The model under review builds one solid part; all positions refer to its coordinate system, in mm. A direction names the side the tool comes from. Give positions to 0.01 mm unless a question says otherwise; leave off trailing zeros. Loops run counter-clockwise (first coordinate to the right, second up) from the corner with the lowest first, then second, coordinate; pieces in that order, holes last. Notation, with made-up numbers: M 16.25,64.5 L 63.25,64.5 A32 ccw 63.25,103.5 Z; hole C 15,61 d11. An arc over 180 degrees is marked long. Put each result on its own line as item: value. Start each with the question number.
from build123d import *

# Parameters (mm, degrees)
SKETCH_1_W                        = 635
SKETCH_1_H                        = 803
SM_BASE_FLANGE_1_DEPTH            = 1
SM_EDGE_FLANGE_1_STRIP_W          = 5.4732
SM_EDGE_FLANGE_1_STRIP_H          = 1
SM_EDGE_FLANGE_1_STRIP_CUT_DEPTH  = 535
SM_EDGE_FLANGE_1_RELIEF_W         = 5.9732
SM_EDGE_FLANGE_1_RELIEF_H         = 0.5
SM_EDGE_FLANGE_1_RELIEF_CUT_DEPTH = 1
SM_EDGE_FLANGE_1_DEPTH            = 535
SM_EDGE_FLANGE_2_STRIP_W          = 5.4732
SM_EDGE_FLANGE_2_STRIP_H          = 1
SM_EDGE_FLANGE_2_STRIP_CUT_DEPTH  = 535
SM_EDGE_FLANGE_2_RELIEF_W         = 5.9732
SM_EDGE_FLANGE_2_RELIEF_H         = 0.5
SM_EDGE_FLANGE_2_RELIEF_CUT_DEPTH = 1
SM_EDGE_FLANGE_2_DEPTH            = 535
SM_EDGE_FLANGE_3_STRIP_W          = 5.4732
SM_EDGE_FLANGE_3_STRIP_H          = 1
SM_EDGE_FLANGE_3_STRIP_CUT_DEPTH  = 703
SM_EDGE_FLANGE_3_RELIEF_W         = 5.9732
SM_EDGE_FLANGE_3_RELIEF_H         = 0.5
SM_EDGE_FLANGE_3_RELIEF_CUT_DEPTH = 1
SM_EDGE_FLANGE_3_DEPTH            = 703
SM_EDGE_FLANGE_3_FLAT_DEPTH       = 1
SKETCH_15_R                       = 3
CUT_EXTRUDE_2_DEPTH               = 752.549898543
SKETCH_16_R                       = 3
CUT_EXTRUDE_3_DEPTH               = 513.258235659


# Sheet-metal steps are written as plain solids
with BuildPart() as part:
    # Sketch 1 → 基体-法兰1 (new body)
    with BuildSketch(Plane.XY):
        Rectangle(SKETCH_1_W, SKETCH_1_H)
    extrude(amount=-SM_BASE_FLANGE_1_DEPTH)

    # 边线-法兰1 strip (across the edge) → 边线-法兰1 strip cut (cut)
    with BuildSketch(Plane(origin=(-267.5, 401.5, -1), x_dir=(0, -1, 0), z_dir=(1, 0, 0))):
        with Locations((-1, -0.5)):
            Rectangle(SM_EDGE_FLANGE_1_STRIP_W, SM_EDGE_FLANGE_1_STRIP_H)
    extrude(amount=SM_EDGE_FLANGE_1_STRIP_CUT_DEPTH, mode=Mode.SUBTRACT)

    # 边线-法兰1 relief (on the sheet) → 边线-法兰1 relief cut (cut)
    with BuildSketch(Plane(origin=(-267.5, 399.7634, -1), x_dir=(0, -1, 0), z_dir=(0, 0, -1))):
        with Locations((-2.4866, 0.25)):
            Rectangle(SM_EDGE_FLANGE_1_RELIEF_W, SM_EDGE_FLANGE_1_RELIEF_H)
        with Locations((-2.4866, -535.25)):
            Rectangle(SM_EDGE_FLANGE_1_RELIEF_W, SM_EDGE_FLANGE_1_RELIEF_H)
    extrude(amount=-SM_EDGE_FLANGE_1_RELIEF_CUT_DEPTH, mode=Mode.SUBTRACT)

    # 边线-法兰1 section (across the edge) → 边线-法兰1 (add)
    with BuildSketch(Plane(origin=(-267.5, 401.5, -1), x_dir=(0, -1, 0), z_dir=(1, 0, 0))):
        with BuildLine():
            Line((0, 0.7366), (0, 19))
            Line((0, 19), (1, 19))
            Line((1, 19), (1, 0.7366))
            ThreePointArc((1, 0.7366), (1.215745145, 0.215745145), (1.7366, 0))
            Line((1.7366, 0), (1.7366, -1))
            ThreePointArc((1.7366, -1), (0.508638364, -0.491361636), (0, 0.7366))
        make_face()
    extrude(amount=SM_EDGE_FLANGE_1_DEPTH)

    # 边线-法兰2 strip (across the edge) → 边线-法兰2 strip cut (cut)
    with BuildSketch(Plane(origin=(267.5, -401.5, -1), x_dir=(0, 1, 0), z_dir=(-1, 0, 0))):
        with Locations((-1, -0.5)):
            Rectangle(SM_EDGE_FLANGE_2_STRIP_W, SM_EDGE_FLANGE_2_STRIP_H)
    extrude(amount=SM_EDGE_FLANGE_2_STRIP_CUT_DEPTH, mode=Mode.SUBTRACT)

    # 边线-法兰2 relief (on the sheet) → 边线-法兰2 relief cut (cut)
    with BuildSketch(Plane(origin=(267.5, -399.7634, -1), x_dir=(0, 1, 0), z_dir=(0, 0, -1))):
        with Locations((-2.4866, 0.25)):
            Rectangle(SM_EDGE_FLANGE_2_RELIEF_W, SM_EDGE_FLANGE_2_RELIEF_H)
        with Locations((-2.4866, -535.25)):
            Rectangle(SM_EDGE_FLANGE_2_RELIEF_W, SM_EDGE_FLANGE_2_RELIEF_H)
    extrude(amount=-SM_EDGE_FLANGE_2_RELIEF_CUT_DEPTH, mode=Mode.SUBTRACT)

    # 边线-法兰2 section (across the edge) → 边线-法兰2 (add)
    with BuildSketch(Plane(origin=(267.5, -401.5, -1), x_dir=(0, 1, 0), z_dir=(-1, 0, 0))):
        with BuildLine():
            Line((0, 0.7366), (0, 19))
            Line((0, 19), (1, 19))
            Line((1, 19), (1, 0.7366))
            ThreePointArc((1, 0.7366), (1.215745145, 0.215745145), (1.7366, 0))
            Line((1.7366, 0), (1.7366, -1))
            ThreePointArc((1.7366, -1), (0.508638364, -0.491361636), (0, 0.7366))
        make_face()
    extrude(amount=SM_EDGE_FLANGE_2_DEPTH)

    # 边线-法兰3 strip (across the edge) → 边线-法兰3 strip cut (cut)
    with BuildSketch(Plane(origin=(317.5, 351.5, -1), x_dir=(-1, 0, 0), z_dir=(0, -1, 0))):
        with Locations((-1, -0.5)):
            Rectangle(SM_EDGE_FLANGE_3_STRIP_W, SM_EDGE_FLANGE_3_STRIP_H)
    sm_edge_flange_3_strip_cut = extrude(amount=SM_EDGE_FLANGE_3_STRIP_CUT_DEPTH, mode=Mode.SUBTRACT)

    # 边线-法兰3 relief (on the sheet) → 边线-法兰3 relief cut (cut)
    with BuildSketch(Plane(origin=(315.7634, 351.5, -1), x_dir=(-1, 0, 0), z_dir=(0, 0, -1))):
        with Locations((-2.4866, 0.25)):
            Rectangle(SM_EDGE_FLANGE_3_RELIEF_W, SM_EDGE_FLANGE_3_RELIEF_H)
        with Locations((-2.4866, -703.25)):
            Rectangle(SM_EDGE_FLANGE_3_RELIEF_W, SM_EDGE_FLANGE_3_RELIEF_H)
    sm_edge_flange_3_relief_cut = extrude(amount=-SM_EDGE_FLANGE_3_RELIEF_CUT_DEPTH, mode=Mode.SUBTRACT)

    # 边线-法兰3 bend section (across the edge) → 边线-法兰3 (add)
    with BuildSketch(Plane(origin=(317.5, 351.5, -1), x_dir=(-1, 0, 0), z_dir=(0, -1, 0))):
        with BuildLine():
            Line((0, 0.7366), (1, 0.7366))
            ThreePointArc((1, 0.7366), (1.215745145, 0.215745145), (1.7366, 0))
            Line((1.7366, 0), (1.7366, -1))
            ThreePointArc((1.7366, -1), (0.508638364, -0.491361636), (0, 0.7366))
        make_face()
    sm_edge_flange_3 = extrude(amount=SM_EDGE_FLANGE_3_DEPTH)

    # 边线-法兰3 profile (on flange) → 边线-法兰3 flat (add)
    with BuildSketch(Plane(origin=(317.5, 0, -1), x_dir=(0, -1, 0), z_dir=(1, 0, 0))):
        Polygon((351.5, 0.7366), (351.5, 19), (87.5, 19), (87.5, 1), (71.5, 1), (71.5, 19), (-351.5, 19), (-351.5, 0.7366), align=None)
    sm_edge_flange_3_flat = extrude(amount=-SM_EDGE_FLANGE_3_FLAT_DEPTH)

    # 镜向1: 边线-法兰3 strip cut, 边线-法兰3 relief cut, 边线-法兰3, 边线-法兰3 flat across plane
    add(sm_edge_flange_3_strip_cut.mirror(Plane(origin=(0, 0, 0), x_dir=(0, 0, 1), z_dir=(1, 0, 0))), mode=Mode.SUBTRACT)
    add(sm_edge_flange_3_relief_cut.mirror(Plane(origin=(0, 0, 0), x_dir=(0, 0, 1), z_dir=(1, 0, 0))), mode=Mode.SUBTRACT)
    add(sm_edge_flange_3.mirror(Plane(origin=(0, 0, 0), x_dir=(0, 0, 1), z_dir=(1, 0, 0))))
    add(sm_edge_flange_3_flat.mirror(Plane(origin=(0, 0, 0), x_dir=(0, 0, 1), z_dir=(1, 0, 0))))

    # 草图15 → 切除-拉伸2 (cut, through all)
    with BuildSketch(Plane(origin=(317.5, 0, 0), x_dir=(0, 0, -1), z_dir=(1, 0, 0))):
        with Locations((10, 321.5)):
            Circle(SKETCH_15_R)
        with Locations((10, 161.5)):
            Circle(SKETCH_15_R)
        with Locations((10, 1.5)):
            Circle(SKETCH_15_R)
        with Locations((10, -158.5)):
            Circle(SKETCH_15_R)
        with Locations((10, -318.5)):
            Circle(SKETCH_15_R)
    extrude(amount=-CUT_EXTRUDE_2_DEPTH, mode=Mode.SUBTRACT)

    # 草图16 → 切除-拉伸3 (cut, through all)
    with BuildSketch(Plane.XY):
        with Locations((308.5, 392.5)):
            Circle(SKETCH_16_R)
        with Locations((308.5, -392.5)):
            Circle(SKETCH_16_R)
        with Locations((-308.5, 392.5)):
            Circle(SKETCH_16_R)
        with Locations((-308.5, -392.5)):
            Circle(SKETCH_16_R)
    extrude(amount=-CUT_EXTRUDE_3_DEPTH, mode=Mode.SUBTRACT)


solid = part.part
(1) We need section A-A, the plane x = -57.5. Write out the cut boundary in (y, z).
(2) To check wall thickness, follow L1, parallel to Y at x = 308.5, z = -0.3; L2, parallel to X at y = -392.5, z = -0.65; L3, parallel to Y at x = -114.5, z = -10.75. State the ranges of each line that lie inside material, in increasing order. Write a range as [from, to].
(3) We need section B-B, the plane z = -10. State how many separate pieces and enclosed holes the cut face has, plus the area to 3 significant figures.
(4) For faces 1 (the flat face through (-4, 400.5, -11)), 2 (the flat face through (-316.5, 5, -11)), 3 (the flat face through (4, -401.5, -11)), list the 3-axis set-ups (+Z, -Z, +X, -X, +Y, -Y) from which the entire face can be reached by the end or side of a thin tool; tool diameter is ignored.
(5) We need section C-C, the plane y = 265. Write out the cut boundary in (x, z).
(6) Insertion check: pin 1 (0.6 mm diameter, centred on y = 351.5, z = -0.5, fed in from +X); pin 2 (2 mm diameter, centred on x = 59.5, y = 250.5, fed in from -Z); pin 3 (2.5 mm diameter, centred on y = -400.5, z = -13.5, fed in from -X). Each pin has a flat end and moves straight along its axis. Give the tip position at first contact, or say it passes through.
(7) Draft analysis for pull direction X (two halves, no side actions). For faces 4 (the flat face through (-4, 6, -1)), 5 (the flat face through (-4, 6, 0)), 6 (the flat face through (-317.5, 5, -11)), state which applies: +X half, -X half, draft (parallel to the pull), parting line (faces both ways), or undercut.
Check sheet entries:
1. outline: M -401.5,-20 L -400.5,-20 L -400.5,-1.74 A0.74 cw -399.76,-1 L 399.76,-1 A0.74 cw 400.5,-1.74 L 400.5,-20 L 401.5,-20 L 401.5,-1.74 A1.74 ccw 399.76,0 L -399.76,0 A1.74 ccw -401.5,-1.74 Z
2. L1: y = [-401.5, -395.5], [-389.5, 389.5], [395.5, 401.5]
2. L2: x = [-317.5, -311.5], [-305.5, 305.5], [311.5, 317.5]
2. L3: y = [-401.5, -400.5], [400.5, 401.5]
3. separate pieces: 16
3. enclosed holes: 0
3. area: 2,380 mm²
4. face 1: -Z, +X, -X
4. face 2: -Z, +Y, -Y
4. face 3: +Z, -Z, +X, -X, -Y
5. outline: M -317.5,-20 L -316.5,-20 L -316.5,-1.74 A0.74 cw -315.76,-1 L 315.76,-1 A0.74 cw 316.5,-1.74 L 316.5,-20 L 317.5,-20 L 317.5,-1.74 A1.74 ccw 315.76,0 L -315.76,0 A1.74 ccw -317.5,-1.74 Z
6. pin 1: stops at x = 317.23
6. pin 2: stops at z = -1
6. pin 3: stops at x = -267.5
7. face 4: undercut
7. face 5: draft
7. face 6: -X half
